Check sheet for the modelled part. Datum: model origin and axes. Units: mm. Coordinates: 2 decimals unless noted, no trailing zeros. Loops run counter-clockwise (first coordinate to the right, second up) from the corner with the lowest first, then second, coordinate; pieces in that order, holes last. Notation, with made-up numbers: (35, -17) - (48, -17) arc R9 ccw to (48, -7) - close; hole circle Ø9 at (38.25, 54.5). An arc over 180 degrees is marked (long way). Use a Markdown table: item, result. Add a question column.
1) Sectioned sample at B-B, the plane y = -14. Enter the section's corners in (x, z) (3 decimals).
2) Sectioned sample at A-A, the plane x = 13.5. Enter the section's corners in (y, z), then the cut area to 3 significant figures.
3) Thickness scan on line 1 (X direction, y = -20.75, z = 55); line 2 (X direction, y = -14, z = 6). Record the ranges inside material, lowest first.
from build123d import *

# Parameters (mm, degrees)
F1_DEPTH = 22.86


with BuildPart() as f1:
    # F0 (on Front) → F1 (new body)
    with BuildSketch(Plane.XZ):
        with BuildLine():
            Line((0, 93.98), (0, 0))
            Line((0, 0), (17.145, 0))
            Line((17.145, 0), (17.145, 3.175))
            ThreePointArc((17.145, 3.175), (11.43, 8.89), (17.145, 14.605))
            Line((17.145, 14.605), (17.145, 18.415))
            ThreePointArc((17.145, 18.415), (11.43, 24.13), (17.145, 29.845))
            Line((17.145, 29.845), (17.145, 33.655))
            ThreePointArc((17.145, 33.655), (11.43, 39.37), (17.145, 45.085))
            Line((17.145, 45.085), (17.145, 48.895))
            ThreePointArc((17.145, 48.895), (11.43, 54.61), (17.145, 60.325))
            Line((17.145, 60.325), (17.145, 64.135))
            ThreePointArc((17.145, 64.135), (11.43, 69.85), (17.145, 75.565))
            Line((17.145, 75.565), (17.145, 79.375))
            ThreePointArc((17.145, 79.375), (11.43, 85.09), (17.145, 90.805))
            Line((17.145, 90.805), (17.145, 93.98))
            Line((17.145, 93.98), (0, 93.98))
        make_face()
        with BuildLine():
            Line((17.145, 3.175), (17.145, 0))
            Line((17.145, 0), (34.29, 0))
            Line((34.29, 0), (34.29, 93.98))
            Line((34.29, 93.98), (17.145, 93.98))
            Line((17.145, 93.98), (17.145, 90.805))
            ThreePointArc((17.145, 90.805), (21.1861152545, 89.1311152545), (22.86, 85.09))
            ThreePointArc((22.86, 85.09), (21.1861152545, 81.0488847455), (17.145, 79.375))
            Line((17.145, 79.375), (17.145, 75.565))
            ThreePointArc((17.145, 75.565), (21.1861152545, 73.8911152545), (22.86, 69.85))
            ThreePointArc((22.86, 69.85), (21.1861152545, 65.8088847455), (17.145, 64.135))
            Line((17.145, 64.135), (17.145, 60.325))
            ThreePointArc((17.145, 60.325), (21.1861152545, 58.6511152545), (22.86, 54.61))
            ThreePointArc((22.86, 54.61), (21.1861152545, 50.5688847455), (17.145, 48.895))
            Line((17.145, 48.895), (17.145, 45.085))
            ThreePointArc((17.145, 45.085), (21.1861152545, 43.4111152545), (22.86, 39.37))
            ThreePointArc((22.86, 39.37), (21.1861152545, 35.3288847455), (17.145, 33.655))
            Line((17.145, 33.655), (17.145, 29.845))
            ThreePointArc((17.145, 29.845), (21.1861152545, 28.1711152545), (22.86, 24.13))
            ThreePointArc((22.86, 24.13), (21.1861152545, 20.0888847455), (17.145, 18.415))
            Line((17.145, 18.415), (17.145, 14.605))
            ThreePointArc((17.145, 14.605), (21.1861152545, 12.9311152545), (22.86, 8.89))
            ThreePointArc((22.86, 8.89), (21.1861152545, 4.8488847455), (17.145, 3.175))
        make_face()
    extrude(amount=F1_DEPTH)


solid = f1.part
Solved:
| question | item | result |
|---|---|---|
| 1 | outline | (0, 0) - (34.29, 0) - (34.29, 93.98) - (0, 93.98) - close; hole circle Ø11.43 at (17.145, 8.89); hole circle Ø11.43 at (17.145, 24.13); hole circle Ø11.43 at (17.145, 39.37); hole circle Ø11.43 at (17.145, 54.61); hole circle Ø11.43 at (17.145, 69.85); hole circle Ø11.43 at (17.145, 85.09) |
| 2 | outline | (-22.86, 0) - (0, 0) - (0, 4.49) - (-22.86, 4.49) - close; (-22.86, 13.29) - (0, 13.29) - (0, 19.73) - (-22.86, 19.73) - close; (-22.86, 28.53) - (0, 28.53) - (0, 34.97) - (-22.86, 34.97) - close; (-22.86, 43.77) - (0, 43.77) - (0, 50.21) - (-22.86, 50.21) - close; (-22.86, 59.01) - (0, 59.01) - (0, 65.45) - (-22.86, 65.45) - close; (-22.86, 74.25) - (0, 74.25) - (0, 80.69) - (-22.86, 80.69) - close; (-22.86, 89.49) - (0, 89.49) - (0, 93.98) - (-22.86, 93.98) - close |
| 2 | area | 941 mm2 |
| 3 | line 1 | x = 0 to 11.44, 22.85 to 34.29 |
| 3 | line 2 | x = 0 to 12.21, 22.08 to 34.29 |
